```python
from build123d import *

# Parameters (mm, degrees)
EXTRUDE_START       = -2
EXTRUDE_1_DEPTH     = 2
CUT_EXTRUDE_1_REACH = 74.196
SKETCH_2_4_R        = 1.55


with BuildPart() as part:
    # Sketch 1 → Revolve 1 (revolve)
    with BuildSketch(Plane.XY, mode=Mode.PRIVATE) as revolve_1_sk:
        Polygon((29, 0), (29, 3.2), (30, 3.2), (30, 1.7), (50, 1.7), (50, 3.2), (51, 3.2), (51, 0), align=None)
    revolve(revolve_1_sk.sketch.rotate(Axis((0, 0, 0), (0, 1, 0)), 90), axis=Axis((0, 0, 0), (0, 1, 0)))

    # Sketch 2 → Extrude 1 (add)
    with BuildSketch(Plane.XZ.offset(EXTRUDE_START)):
        with BuildLine():
            Line((-3.05, 26), (-3.05, 28.839166077))
            ThreePointArc((-3.05, 28.839166077), (0, 29), (3.05, 28.839166077))
            Line((3.05, 28.839166077), (3.05, 26))
            ThreePointArc((3.05, 26), (0, 22.95), (-3.05, 26))
        make_face()
        with BuildLine():
            Line((26, 3.05), (28.839166077, 3.05))
            ThreePointArc((28.839166077, 3.05), (29, 0), (28.839166077, -3.05))
            Line((28.839166077, -3.05), (26, -3.05))
            ThreePointArc((26, -3.05), (22.95, 0), (26, 3.05))
        make_face()
        with BuildLine():
            Line((3.05, -26), (3.05, -28.839166077))
            ThreePointArc((3.05, -28.839166077), (0, -29), (-3.05, -28.839166077))
            Line((-3.05, -28.839166077), (-3.05, -26))
            ThreePointArc((-3.05, -26), (0, -22.95), (3.05, -26))
        make_face()
        with BuildLine():
            Line((-26, -3.05), (-28.839166077, -3.05))
            ThreePointArc((-28.839166077, -3.05), (-29, 0), (-28.839166077, 3.05))
            Line((-28.839166077, 3.05), (-26, 3.05))
            ThreePointArc((-26, 3.05), (-22.95, 0), (-26, -3.05))
        make_face()
    extrude(amount=EXTRUDE_1_DEPTH)

    # Sketch 2_4 → Cut-Extrude 1 (cut, up to next)
    with BuildSketch(Plane.XZ, mode=Mode.PRIVATE) as cut_extrude_1_sk1:
        with Locations(Location((0, 26, 0), (0, 0, 270))):
            Circle(SKETCH_2_4_R)
    cut_extrude_1_tool1 = extrude(cut_extrude_1_sk1.sketch, amount=-CUT_EXTRUDE_1_REACH, mode=Mode.PRIVATE) & part.part
    # Sketch 2_4 → Cut-Extrude 1 (cut, up to next)
    with BuildSketch(Plane.XZ, mode=Mode.PRIVATE) as cut_extrude_1_sk2:
        with Locations(Location((26, 0, 0), (0, 0, 270))):
            Circle(SKETCH_2_4_R)
    cut_extrude_1_tool2 = extrude(cut_extrude_1_sk2.sketch, amount=-CUT_EXTRUDE_1_REACH, mode=Mode.PRIVATE) & part.part
    # Sketch 2_4 → Cut-Extrude 1 (cut, up to next)
    with BuildSketch(Plane.XZ, mode=Mode.PRIVATE) as cut_extrude_1_sk3:
        with Locations(Location((0, -26, 0), (0, 0, 270))):
            Circle(SKETCH_2_4_R)
    cut_extrude_1_tool3 = extrude(cut_extrude_1_sk3.sketch, amount=-CUT_EXTRUDE_1_REACH, mode=Mode.PRIVATE) & part.part
    # Sketch 2_4 → Cut-Extrude 1 (cut, up to next)
    with BuildSketch(Plane.XZ, mode=Mode.PRIVATE) as cut_extrude_1_sk4:
        with Locations(Location((-26, 0, 0), (0, 0, 270))):
            Circle(SKETCH_2_4_R)
    cut_extrude_1_tool4 = extrude(cut_extrude_1_sk4.sketch, amount=-CUT_EXTRUDE_1_REACH, mode=Mode.PRIVATE) & part.part
    add(cut_extrude_1_tool1.solids().sort_by_distance((0, 0, 26))[0], mode=Mode.SUBTRACT)
    add(cut_extrude_1_tool2.solids().sort_by_distance((26, 0, 0))[0], mode=Mode.SUBTRACT)
    add(cut_extrude_1_tool3.solids().sort_by_distance((0, 0, -26))[0], mode=Mode.SUBTRACT)
    add(cut_extrude_1_tool4.solids().sort_by_distance((-26, 0, 0))[0], mode=Mode.SUBTRACT)


solid = part.part
```
Input: part model. Units: mm. Frame: model coordinates. A direction names the side the tool comes from. Give positions to 0.01 mm unless a question says otherwise; leave off trailing zeros. Order: outer loops, then holes, each group sorted by start corner. A loop starts at its lowest first (then second) coordinate and runs counter-clockwise, first axis right, second up. Notation, with made-up numbers: M 25,82 L 64,82 A14 ccw 64,98 Z; hole C 73,-10.75 d1. An arc over 180 degrees is marked long. One line per question, with ' | ' between items. Start each with the question number.
1. Section query B-B (y = 0.6). Return the cut outline in (x, z), and give its area (3 significant figures).
2. Access query for faces 1 (the face through (0.07, 1.01, 22.95)), 2 (the face through (-25, 3.2, -16)), 3 (the face through (-28, 2, 0)). Directions: +Z, -Z, +X, -X, +Y, -Y. A direction counts if a zero-diameter tool reaches every point of the face in a straight line with its end or side. Return the directions, or none.
3. Material intervals for probe 1 along X at (y, z) = (2, 16); probe 2 along X at (y, z) = (2.9, -3); probe 3 along X at (y, z) = (1.9, -25), sorted ascending. Write a range as [from, to].
4. Section query D-D (z = -19.5). Return the cut outline in (x, y).
5. Section query C-C (x = 0). Return the cut outline in (y, z).
6. Pull-direction query (X, two-part tool) for faces 4 (the face through (31.033, 1.578, 40.472)), 5 (the face through (27.4, 2, -1.3)), 6 (the face through (37.5, 3.2, 33.8)); classes: released by +X, released by -X, zero draft, split by the parting line, or undercut.
7. First-contact query: pin 1 Ø3.5 at (x, z) = (-26, 0) entering from -Y; pin 2 Ø1.9 at (x, z) = (0, 26) entering from -Y; pin 3 Ø1.6 at (x, y) = (-27, 1.5) entering from -Z; pin 4 Ø6.5 at (x, z) = (25, -1) entering from +Y. Flat tips, straight axial feed; report the tip coordinate or a pass-through.
8. Section query A-A (z = 0). Return the cut outline in (x, y).
Here are the results:
1) outline: C 0,0 d102; hole M -28.84,-3.05 A29 ccw -3.05,-28.84 L -3.05,-26 A3.05 cw 3.05,-26 L 3.05,-28.84 A29 ccw 28.84,-3.05 L 26,-3.05 A3.05 cw 26,3.05 L 28.84,3.05 A29 ccw 3.05,28.84 L 3.05,26 A3.05 cw -3.05,26 L -3.05,28.84 A29 ccw -28.84,3.05 L -26,3.05 A3.05 cw -26,-3.05 Z; hole C -26,0 d3.1; hole C 0,-26 d3.1; hole C 0,26 d3.1; hole C 26,0 d3.1 | area: 5,630 mm²
2) face 1: +Y, -Y | face 2: +Z, -Z, +X, -X, +Y | face 3: +Y
3) probe 1: [-48.43, -47.37], [-25.38, -24.19], [24.19, 25.38], [47.37, 48.43] | probe 2: [-50.91, -49.91], [-29.85, -28.84], [28.84, 29.85], [49.91, 50.91] | probe 3: [-44.45, -43.3], [-16.58, -14.7], [-2.88, -1.18], [1.18, 2.88], [14.7, 16.58], [43.3, 44.45]
4) outline: M -47.12,0 L -21.47,0 L -21.47,3.2 L -22.8,3.2 L -22.8,1.7 L -46.04,1.7 L -46.04,3.2 L -47.12,3.2 Z; M 21.47,0 L 47.12,0 L 47.12,3.2 L 46.04,3.2 L 46.04,1.7 L 22.8,1.7 L 22.8,3.2 L 21.47,3.2 Z
5) outline: M 0,-51 L 3.2,-51 L 3.2,-50 L 1.7,-50 L 1.7,-30 L 3.2,-30 L 3.2,-29 L 2,-29 L 2,-27.55 L 0,-27.55 Z; M 0,-24.45 L 2,-24.45 L 2,-22.95 L 0,-22.95 Z; M 0,22.95 L 2,22.95 L 2,24.45 L 0,24.45 Z; M 0,27.55 L 2,27.55 L 2,29 L 3.2,29 L 3.2,30 L 1.7,30 L 1.7,50 L 3.2,50 L 3.2,51 L 0,51 Z
6) face 4: split by the parting line | face 5: undercut | face 6: zero draft
7) pin 1: y = 0 | pin 2: through | pin 3: z = -43.76 | pin 4: y = 2
8) outline: M -51,0 L -27.55,0 L -27.55,2 L -29,2 L -29,3.2 L -30,3.2 L -30,1.7 L -50,1.7 L -50,3.2 L -51,3.2 Z; M -24.45,0 L -22.95,0 L -22.95,2 L -24.45,2 Z; M 22.95,0 L 24.45,0 L 24.45,2 L 22.95,2 Z; M 27.55,0 L 51,0 L 51,3.2 L 50,3.2 L 50,1.7 L 30,1.7 L 30,3.2 L 29,3.2 L 29,2 L 27.55,2 Z
